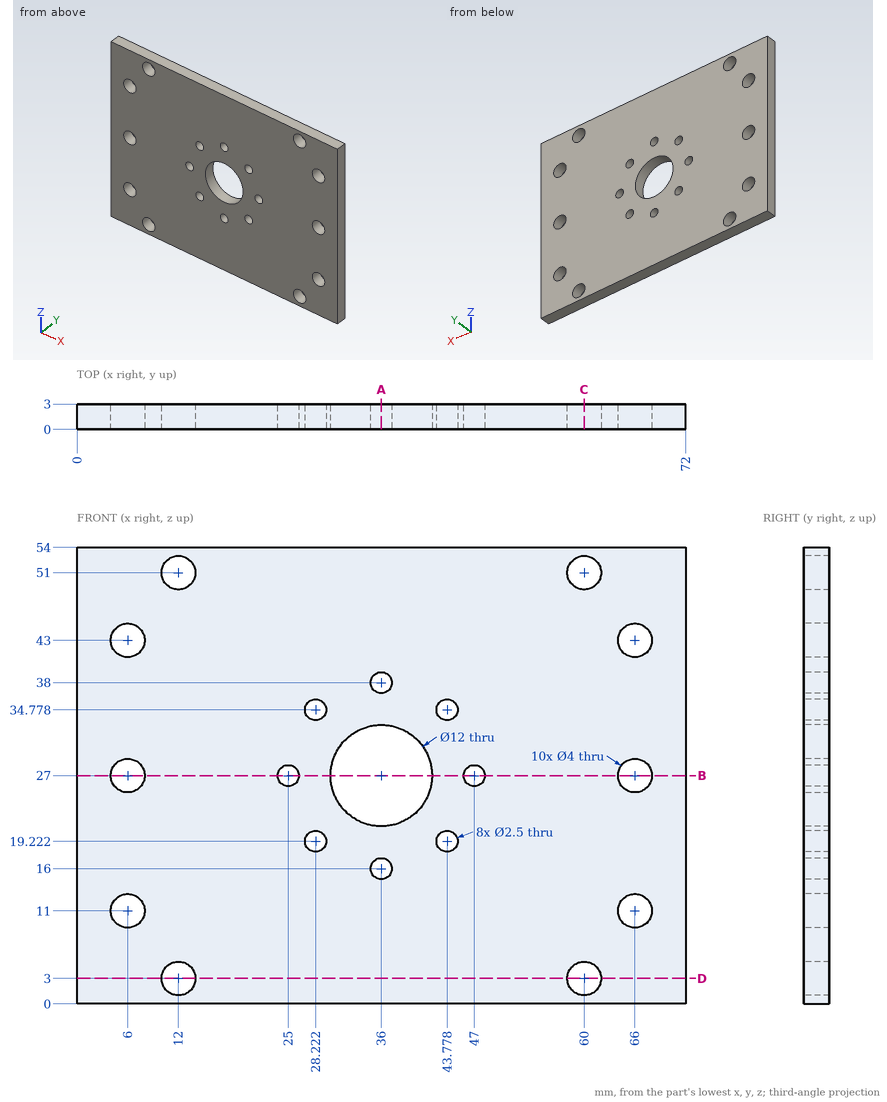
Job drawing, mm, ordinate dimensions from the low corner. One solid piece. Round coordinates to 2 decimals unless told otherwise and drop trailing zeros. Loops run counter-clockwise (first coordinate to the right, second up) from the corner with the lowest first, then second, coordinate; pieces in that order, holes last.
Item 1: Cut at D-D, the plane z = 3. Give the cut face in (x, y), then the cut area to 3 significant figures.
Item 2: Cut at B-B, the plane z = 27. Give the cut face in (x, y).
Item 3: Cut at A-A, the plane x = 36. Give the cut face in (y, z), then the cut area to 3 significant figures.
Item 4: Drop flat-ended pins along their axis: P1, Ø1.5, axis at x = 36, z = 16, coming from the -Y side; P2, Ø4.5, axis at x = 6, z = 43, coming from the +Y side. Give the stop position or say it passes through.
Item 5: Drill centre lines: line 1 (Z direction, x = 66, y = 0.9); line 2 (Z direction, x = 36, y = 1.15); line 3 (Z direction, x = 61.5, y = 0.3). Where is each one in solid material? Low to high.
Item 6: Cut at C-C, the plane x = 60. Give the cut face in (y, z).
A:
1. outline: (0, 0) - (10, 0) - (10, 3) - (0, 3) - close; (14, 0) - (58, 0) - (58, 3) - (14, 3) - close; (62, 0) - (72, 0) - (72, 3) - (62, 3) - close
1. area: 192 mm2
2. outline: (0, 0) - (4, 0) - (4, 3) - (0, 3) - close; (8, 0) - (23.75, 0) - (23.75, 3) - (8, 3) - close; (26.25, 0) - (30, 0) - (30, 3) - (26.25, 3) - close; (42, 0) - (45.75, 0) - (45.75, 3) - (42, 3) - close; (48.25, 0) - (64, 0) - (64, 3) - (48.25, 3) - close; (68, 0) - (72, 0) - (72, 3) - (68, 3) - close
3. outline: (0, 0) - (3, 0) - (3, 14.75) - (0, 14.75) - close; (0, 17.25) - (3, 17.25) - (3, 21) - (0, 21) - close; (0, 33) - (3, 33) - (3, 36.75) - (0, 36.75) - close; (0, 39.25) - (3, 39.25) - (3, 54) - (0, 54) - close
3. area: 111 mm2
4. P1: passes through
4. P2: stops at y = 3
5. line 1: z = 0 to 9, 13 to 25, 29 to 41, 45 to 54
5. line 2: z = 0 to 14.75, 17.25 to 21, 33 to 36.75, 39.25 to 54
5. line 3: z = 0 to 1.68, 4.32 to 49.68, 52.32 to 54
6. outline: (0, 0) - (3, 0) - (3, 1) - (0, 1) - close; (0, 5) - (3, 5) - (3, 49) - (0, 49) - close; (0, 53) - (3, 53) - (3, 54) - (0, 54) - close
